from build123d import *

# Parameters (mm, degrees)
F0_R     = 40
F0_R_2   = 2.5
F1_DEPTH = 10


with BuildPart() as f1:
    # F0 (on Front) → F1 (new body)
    with BuildSketch(Plane.XZ):
        Circle(F0_R)
        with BuildLine():
            ThreePointArc((-5.59017, -5), (-5.303301, -5.303301), (-5, -5.59017))
            Line((-5, -5.59017), (-5, -32.113081))
            ThreePointArc((-5, -32.113081), (-22.98097, -22.98097), (-32.113081, -5))
            Line((-32.113081, -5), (-5.59017, -5))
        make_face(mode=Mode.SUBTRACT)
        with BuildLine():
            Line((5.59017, -5), (32.113081, -5))
            ThreePointArc((32.113081, -5), (22.98097, -22.98097), (5, -32.113081))
            Line((5, -32.113081), (5, -5.59017))
            ThreePointArc((5, -5.59017), (5.303301, -5.303301), (5.59017, -5))
        make_face(mode=Mode.SUBTRACT)
        with BuildLine():
            ThreePointArc((-32.113081, 5), (-22.98097, 22.98097), (-5, 32.113081))
            Line((-5, 32.113081), (-5, 5.59017))
            ThreePointArc((-5, 5.59017), (-5.303301, 5.303301), (-5.59017, 5))
            Line((-5.59017, 5), (-32.113081, 5))
        make_face(mode=Mode.SUBTRACT)
        Circle(F0_R_2, mode=Mode.SUBTRACT)
        with BuildLine():
            Line((32.113081, 5), (5.59017, 5))
            ThreePointArc((5.59017, 5), (5.303301, 5.303301), (5, 5.59017))
            Line((5, 5.59017), (5, 32.113081))
            ThreePointArc((5, 32.113081), (22.98097, 22.98097), (32.113081, 5))
        make_face(mode=Mode.SUBTRACT)
    extrude(amount=F1_DEPTH)


solid = f1.part
Build history of the part. All positions in model axes, mm. A direction names the side the tool comes from. Give positions to 0.01 mm unless a question says otherwise; leave off trailing zeros. Order: outer loops, then holes, each group sorted by start corner. A loop starts at its lowest first (then second) coordinate and runs counter-clockwise, first axis right, second up. Notation, with made-up numbers: M 9.25,37 L 33.25,37 A23 cw 33.25,55 Z; hole C 86,-40 d3. An arc over 180 degrees is marked long. Put each result on its own line as item: value.
Item 1: Slice it at C-C, the plane y = -3. Write the cut outline in (x, z), plus the area to 3 significant figures.
From the geometry:
outline: C 0,0 d80; hole M -32.11,-5 A32.5 ccw -5,-32.11 L -5,-5.59 A7.5 cw -5.59,-5 Z; hole M -32.11,5 L -5.59,5 A7.5 cw -5,5.59 L -5,32.11 A32.5 ccw Z; hole C 0,0 d5; hole M 5,-32.11 A32.5 ccw 32.11,-5 L 5.59,-5 A7.5 cw 5,-5.59 Z; hole M 5,5.59 A7.5 cw 5.59,5 L 32.11,5 A32.5 ccw 5,32.11 Z
area: 2,880 mm2
Item 2: Slice it at D-D, the plane z = 10. Write the cut outline in (x, y), plus the area to 3 significant figures.
From the geometry:
outline: M -38.73,-10 L -30.92,-10 L -30.92,0 L -38.73,0 Z; M -5,-10 L 5,-10 L 5,0 L -5,0 Z; M 30.92,-10 L 38.73,-10 L 38.73,0 L 30.92,0 Z
area: 256 mm2
Item 3: Slice it at B-B, the plane z = 0. Write the cut outline in (x, y), plus the area to 3 significant figures.
From the geometry:
outline: M -40,-10 L -2.5,-10 L -2.5,0 L -40,0 Z; M 2.5,-10 L 40,-10 L 40,0 L 2.5,0 Z
area: 750 mm2
Item 4: Probe line 1 (Z direction, x = -28.5, y = -9); line 2 (Z direction, x = 0, y = -8); line 3 (Z direction, x = -25, y = -1.5). List the from-to ranges inside material, lowest first. Write a range as [from, to].
From the geometry:
line 1: z = [-28.07, -15.62], [-5, 5], [15.62, 28.07]
line 2: z = [-40, -2.5], [2.5, 40]
line 3: z = [-31.22, -20.77], [-5, 5], [20.77, 31.22]
Item 5: Slice it at A-A, the plane x = 0. Write the cut outline in (y, z), plus the area to 3 significant figures.
From the geometry:
outline: M -10,-40 L 0,-40 L 0,-2.5 L -10,-2.5 Z; M -10,2.5 L 0,2.5 L 0,40 L -10,40 Z
area: 750 mm2
Item 6: Flat gauge pins, fed straight in: pin 1 Ø2 at (x, y) = (-3.5, -1.5) entering from -Z; pin 2 Ø5 at (y, z) = (-5.5, 25) entering from -X; pin 3 Ø3 at (y, z) = (-7, 21.5) entering from -X; pin 4 Ø3 at (x, z) = (25, 30.5) entering from +Y. Where does each tip first touch, or does it go through?
From the geometry:
pin 1: stops at z = -39.92
pin 2: stops at x = -33.07
pin 3: stops at x = -34.64
pin 4: stops at y = 0
Item 7: Two-plate mould, pull along Z, no slides. Class faces 3 (the flat face through (-19, -5, -5)), 4 (the flat face through (-1, 0, -8)), 5 (the cylindrical face through (-8.67, -4.93, -39.05)): +Z half, -Z half, draft (parallel to the pull), parting line (faces both ways), or undercut.
From the geometry:
face 3: undercut
face 4: draft
face 5: parting line
Item 8: 3-axis set-ups, long thin cutter, end or side, ignore diameter. For faces 1 (the flat face through (5, -5, 19)), 2 (the flat face through (-1, -10, -8)): which of +Z, -Z, +X, -X, +Y, -Y reach the whole face in a straight line?
From the geometry:
face 1: +Y, -Y
face 2: +Z, -Z, +X, -X, -Y
